Could you check a few things on this drawing? It's one solid part, dimensions in mm from its lowest x, y, z. Give positions to 0.01 mm unless a question says otherwise; leave off trailing zeros. Order: outer loops, then holes, each group sorted by start corner. A loop starts at its lowest first (then second) coordinate and runs counter-clockwise, first axis right, second up.
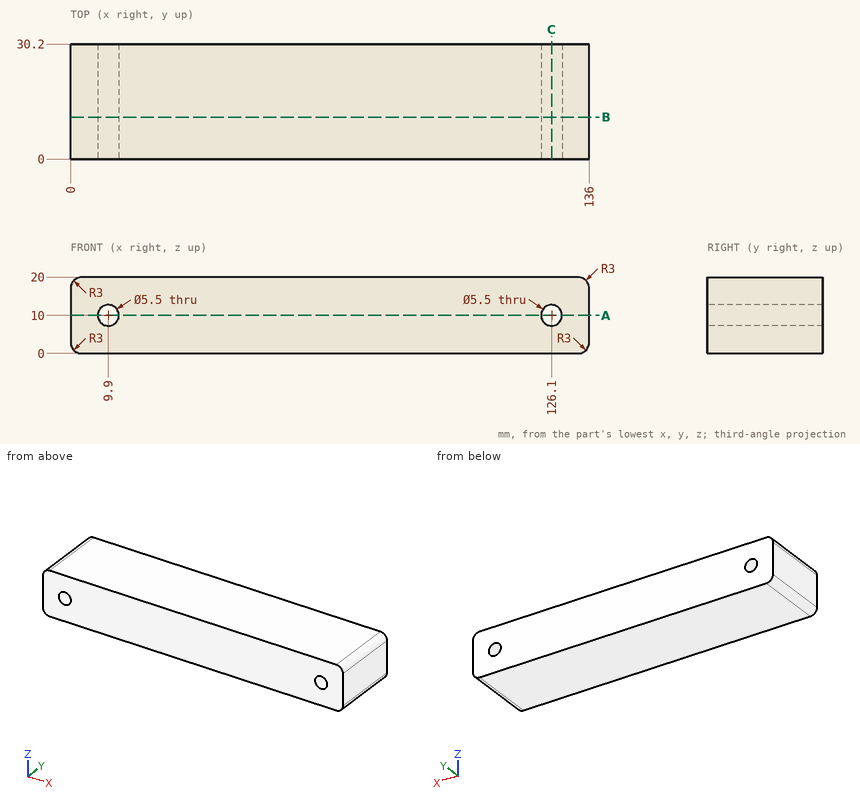
1) If I drill on line 1 (X direction, y = 9, z = 9.75); line 2 (Z direction, x = 126.1, y = 15); line 3 (X direction, y = 19.5, z = 12), over which ranges is the centre line in solid material (lowest first)?
2) Suppose I cut it at A-A (z = 10). Please give me the cut outline in (x, y).
3) Suppose I cut it at B-B (y = 11). Please give me the cut outline in (x, z), and give its area (3 significant figures).
4) Suppose I cut it at C-C (x = 126.1). Please give me the cut outline in (y, z).
Results:
1. line 1: x = 0 to 7.16, 12.64 to 123.36, 128.84 to 136
1. line 2: z = 0 to 7.25, 12.75 to 20
1. line 3: x = 0 to 8.01, 11.79 to 124.21, 127.99 to 136
2. outline: (0, 0) - (7.15, 0) - (7.15, 30.2) - (0, 30.2) - close; (12.65, 0) - (123.35, 0) - (123.35, 30.2) - (12.65, 30.2) - close; (128.85, 0) - (136, 0) - (136, 30.2) - (128.85, 30.2) - close
3. outline: (0, 3) arc R3 ccw to (3, 0) - (133, 0) arc R3 ccw to (136, 3) - (136, 17) arc R3 ccw to (133, 20) - (3, 20) arc R3 ccw to (0, 17) - close; hole circle Ø5.5 at (9.9, 10); hole circle Ø5.5 at (126.1, 10)
3. area: 2,660 mm2
4. outline: (0, 0) - (30.2, 0) - (30.2, 7.25) - (0, 7.25) - close; (0, 12.75) - (30.2, 12.75) - (30.2, 20) - (0, 20) - close
